from build123d import *

# Parameters (mm, degrees)
F1_DEPTH = 63.5
F0_W     = 25.4
F0_H     = 19.05
F2_DEPTH = 25.4
F3_DEPTH = 7.9375
F5_R     = 5.08
F6_R     = 5.08
F7_R     = 5.08
F8_R     = 5.08


with BuildPart() as f1:
    # F0 (on Front) → F1 (new body, symmetric)
    with BuildSketch(Plane.XZ):
        Polygon((41.275, -9.525), (41.275, 9.525), (22.225, 9.525), (-41.275, 9.525), (-41.275, -9.525), align=None)
    extrude(amount=F1_DEPTH, both=True)

    # F0 (on Front) → F2 (join, symmetric)
    with BuildSketch(Plane.XZ):
        with BuildLine():
            Line((22.225, 9.525), (41.275, 9.525))
            Line((41.275, 9.525), (41.275, 27.2120934423))
            ThreePointArc((41.275, 27.2120934423), (45.0451659726, 37.4828586606), (54.5649046512, 42.8752))
            Line((54.5649046512, 42.8752), (60.325, 42.8752))
            Line((60.325, 42.8752), (60.325, 61.9252))
            Line((60.325, 61.9252), (53.3086645403, 61.9252))
            ThreePointArc((53.3086645403, 61.9252), (31.1316001075, 50.5101296693), (22.225, 27.2120934423))
            Line((22.225, 27.2120934423), (22.225, 9.525))
        make_face()
        with Locations((73.025, 52.4002)):
            Rectangle(F0_W, F0_H)
    extrude(amount=F2_DEPTH, both=True)

    # F0 (on Front) → F3 (join, symmetric)
    with BuildSketch(Plane.XZ):
        with BuildLine():
            Line((-41.275, 9.525), (22.225, 9.525))
            Line((22.225, 9.525), (22.225, 27.2120934423))
            ThreePointArc((22.225, 27.2120934423), (31.1316001075, 50.5101296693), (53.3086645403, 61.9252))
            add(Edge.make_bspline(
                [(-41.275, 9.525), (-40.7104454935, 50.98317191), (6.0875406489, 61.2558983266), (53.3086645403, 61.9252)],
                knots=[0, 0, 0, 0, 108.1288608925, 108.1288608925, 108.1288608925, 108.1288608925], degree=3))
        make_face()
    extrude(amount=F3_DEPTH, both=True)

    # F0 (on Front) → F4 (revolve)
    with BuildSketch(Plane.XZ):
        Polygon((85.725, 61.9252), (85.725, 42.8752), (85.725, 38.1), (111.125, 38.1), (111.125, 66.675), (85.725, 66.675), align=None)
    revolve(axis=Axis((85.725, 0, 52.3875), (0, 0, 1)))

    # F5
    f5_edges = [f1.edges().sort_by_distance(p)[0] for p in [
        (41.275, -63.5, 0),
    ]]
    fillet(f5_edges, radius=F5_R)

    # F6
    f6_edges = [f1.edges().sort_by_distance(p)[0] for p in [
        (41.275, 63.5, 0),
    ]]
    fillet(f6_edges, radius=F6_R)

    # F7
    f7_edges = [f1.edges().sort_by_distance(p)[0] for p in [
        (-41.275, 63.5, 0),
    ]]
    fillet(f7_edges, radius=F7_R)

    # F8
    f8_edges = [f1.edges().sort_by_distance(p)[0] for p in [
        (-41.275, -63.5, 0),
    ]]
    fillet(f8_edges, radius=F8_R)


solid = f1.part
Design review of the part built by this model. Coordinates are the model's own, in mm. A direction names the side the tool comes from. Coordinates: 2 decimals unless noted, no trailing zeros. Order: outer loops, then holes, each group sorted by start corner. A loop starts at its lowest first (then second) coordinate and runs counter-clockwise, first axis right, second up. Notation, with made-up numbers: (-23, 22.5) -> (33, 22.5) arc R23 cw to (33, 49.5) -> close; hole circle Ø8 at (43, -34). An arc over 180 degrees is marked (long way). One line per item, written item: value.
1) Machinability: for faces 1 (the face through (59, 0, 61.925)), 2 (the face through (31.371, -16.791, 50.775)), 3 (the face through (86, 0, 38.1)), 4 (the face through (44.94, -0.36, 37.36)), which of the approach directions +Z, -Z, +X, -X, +Y, -Y give a long, thin tool a straight path to every point of the face, cutting with its end or side? Answer none if there is none.
Output values:
face 1: +Z, -X
face 2: +Z, -X, -Y
face 3: -Z, +X, +Y, -Y
face 4: -Z, +Y, -Y
2) Draft analysis for pull direction X (two halves, no side actions). For faces 5 (the face through (60, 0, 42.875)), 6 (the face through (-41.275, -1, 0)), 7 (the face through (46, 25.4, 42)), state which applies: +X half, -X half, draft (parallel to the pull), parting line (faces both ways), or undercut.
Output values:
face 5: undercut
face 6: -X half
face 7: draft
3) We need section D-D, the plane y = -55. Give the boundary of the cut face in (x, z) (3 decimals).
Output values:
outline: (-41.275, -9.525) -> (41.275, -9.525) -> (41.275, 9.525) -> (-41.275, 9.525) -> close
4) We need section C-C, the plane y = 18.5. Give the boundary of the cut face in (x, z) (3 decimals), then the cut area to 3 significant figures.
Output values:
outline: (-41.275, -9.525) -> (41.275, -9.525) -> (41.275, 27.212) arc R15.875 cw to (54.565, 42.875) -> (68.321, 42.875) -> (68.321, 38.1) -> (103.129, 38.1) -> (103.129, 66.675) -> (68.321, 66.675) -> (68.321, 61.925) -> (53.309, 61.925) arc R34.925 ccw to (22.225, 27.212) -> (22.225, 9.525) -> (-41.275, 9.525) -> close
area: 3,880 mm2
5) We need section B-B, the plane x = 64.5. Give the boundary of the cut face in (y, z) (3 decimals).
Output values:
outline: (-25.4, 42.875) -> (-13.952, 42.875) -> (-13.952, 38.1) -> (13.952, 38.1) -> (13.952, 42.875) -> (25.4, 42.875) -> (25.4, 61.925) -> (13.952, 61.925) -> (13.952, 66.675) -> (-13.952, 66.675) -> (-13.952, 61.925) -> (-25.4, 61.925) -> close
6) We need section A-A, the plane y = -18. Give the boundary of the cut face in (x, z) (3 decimals).
Output values:
outline: (-41.275, -9.525) -> (41.275, -9.525) -> (41.275, 27.212) arc R15.875 cw to (54.565, 42.875) -> (67.804, 42.875) -> (67.804, 38.1) -> (103.646, 38.1) -> (103.646, 66.675) -> (67.804, 66.675) -> (67.804, 61.925) -> (53.309, 61.925) arc R34.925 ccw to (22.225, 27.212) -> (22.225, 9.525) -> (-41.275, 9.525) -> close
7) Clearance check with flat-ended pins moving along their axes: P1, Ø5, axis at y = 18, z = 19.5, coming from the -X side (3 decimals); P2, Ø25, axis at x = 63.5, y = 0, coming from the -Z side; P3, Ø6, axis at y = -8.5, z = 49.5, coming from the -X side. State where each tip first meets the part, or that it passes through.
Output values:
P1: stops at x = 22.225
P2: stops at z = 38.1
P3: stops at x = -19.99
8) To check wall thickness, follow probe 1 along X at (y, z) = (-42.5, -5.5) (3 decimals); probe 2 along Z at (x, y) = (82.5, 22.5) (3 decimals); probe 3 along Y at (x, z) = (11.5, 11). State the ranges of each line that lie inside material, in increasing order. Write a range as [from, to].
Output values:
probe 1: x = [-41.275, 41.275]
probe 2: z = [38.1, 66.675]
probe 3: y = [-7.94, 7.94]
